```python
from build123d import *


with BuildPart() as f1:
    # F0 (on Front) → F1 (revolve)
    with BuildSketch(Plane.XZ):
        with BuildLine():
            Line((0, 7.565121), (0, 0))
            Line((0, 0), (39.313756, 0))
            Line((39.313756, 0), (51.177312, -21.120233))
            Line((51.177312, -21.120233), (66.577177, -21.120233))
            ThreePointArc((66.577177, -21.120233), (71.067305, -19.260362), (72.927177, -14.770233))
            Line((72.927177, -14.770233), (72.927177, 69.339424))
            Line((72.927177, 69.339424), (56.120466, 87.134771))
            Line((56.120466, 87.134771), (56.120466, 107.401684))
            Line((56.120466, 107.401684), (50.587501, 107.401684))
            Line((50.587501, 107.401684), (50.587501, 82.146585))
            Line((50.587501, 82.146585), (68.7396, 63.994482))
            Line((68.7396, 63.994482), (68.7396, -9.366923))
            ThreePointArc((68.7396, -9.366923), (66.879729, -13.857051), (62.3896, -15.716923))
            Line((62.3896, -15.716923), (56.120466, -15.716923))
            Line((56.120466, -15.716923), (43.484502, 7.565121))
            Line((43.484502, 7.565121), (0, 7.565121))
        make_face()
    revolve(axis=Axis((0, 0, 35.899226), (0, 0, 1)))


solid = f1.part
```
Geometry check sheet. Reference: the model listing, model coordinates, mm. A direction names the side the tool comes from. Give positions to 0.01 mm unless a question says otherwise; leave off trailing zeros. Write each loop counter-clockwise with the first axis right and the second up, starting at its lowest first coordinate (ties: lowest second). Pieces come first, ordered by that corner, then holes. Notation, with made-up numbers: (30, -12.75) - (77, -12.75) arc R30 ccw to (77, 26.25) - close; hole circle Ø1 at (47, 52). An arc over 180 degrees is marked (long way). Use a Markdown table: item, result.
Q1. Section check D-D, the plane z = 46. Enter the section's corners in (x, y), then the cut area to 3 significant figures.
Computed:
| item | result |
|---|---|
| outline | circle Ø145.85 at (0, 0); hole circle Ø137.48 at (0, 0) |
| area | 1,860 mm² |
Q2. Go/stop test with flat-tipped pins: P1, Ø3, axis at x = 48, y = 56, coming from the +Z side; P2, Ø4, axis at x = 38.5, y = -30, coming from the +Z side; P3, Ø5, axis at x = -13.5, y = 35.5, coming from the -Z side; P4, Ø2, axis at x = -25, y = -20.5, coming from the +Z side. Record where each tip stops, or that it passes through.
Computed:
| item | result |
|---|---|
| P1 | stops at z = 70.05 |
| P2 | stops at z = 107.4 |
| P3 | stops at z = -2.08 |
| P4 | stops at z = 7.57 |
Q3. Thickness scan on L1, parallel to Y at x = 0, z = 97.25; L2, parallel to Y at x = 0, z = 33; L3, parallel to Z at x = 1, y = 17.5. Record the ranges inside material, lowest first. Write a range as [from, to].
Computed:
| item | result |
|---|---|
| L1 | y = [-56.12, -50.59], [50.59, 56.12] |
| L2 | y = [-72.93, -68.74], [68.74, 72.93] |
| L3 | z = [0, 7.57] |
Q4. Section check A-A, the plane x = 0. Enter the section's corners in (y, z), then the cut area to 3 significant figures.
Computed:
| item | result |
|---|---|
| outline | (-72.93, -14.77) arc R6.35 ccw to (-66.58, -21.12) - (-51.18, -21.12) - (-39.31, 0) - (39.31, 0) - (51.18, -21.12) - (66.58, -21.12) arc R6.35 ccw to (72.93, -14.77) - (72.93, 69.34) - (56.12, 87.13) - (56.12, 107.4) - (50.59, 107.4) - (50.59, 82.15) - (68.74, 63.99) - (68.74, -9.37) arc R6.35 cw to (62.39, -15.72) - (56.12, -15.72) - (43.48, 7.57) - (-43.48, 7.57) - (-56.12, -15.72) - (-62.39, -15.72) arc R6.35 cw to (-68.74, -9.37) - (-68.74, 63.99) - (-50.59, 82.15) - (-50.59, 107.4) - (-56.12, 107.4) - (-56.12, 87.13) - (-72.93, 69.34) - close |
| area | 2,490 mm² |
Q5. Draft check along Y on faces 4 (the face through (-9, 50, 107.402)), 5 (the face through (-10.966, -49.385, 94.597)), 6 (the face through (38.206, 12.032, -1.321)), 7 (the face through (-72.857, 3.206, 27.873)). Enter one of: pulls with the +Y half, pulls with the -Y half, needs draft (parallel to the pull), parting line crosses it, or undercut.
Computed:
| item | result |
|---|---|
| face 4 | needs draft |
| face 5 | undercut |
| face 6 | undercut |
| face 7 | parting line crosses it |
Q6. Set-up check for faces 1 (the face through (-1, 1, 7.565)), 2 (the face through (42.062, 13.246, 6.435)), 3 (the face through (1, 1, 0)): record each of +Z, -Z, +X, -X, +Y, -Y from which the full face is reachable in a straight line by a thin tool's end or side.
Computed:
| item | result |
|---|---|
| face 1 | +Z |
| face 2 | none |
| face 3 | -Z |
Q7. Section check C-C, the plane z = 96.5. Enter the section's corners in (x, y) (1 decimal).
Computed:
| item | result |
|---|---|
| outline | circle Ø112.2 at (0, 0); hole circle Ø101.2 at (0, 0) |
